The drawing under review shows one solid part. Ordinate dimensions are in mm from its lowest x, y, z. Coordinates: 2 decimals unless noted, no trailing zeros. Order: outer loops, then holes, each group sorted by start corner. A loop starts at its lowest first (then second) coordinate and runs counter-clockwise, first axis right, second up. Notation, with made-up numbers: (60.5, 56.5) - (82.5, 56.5) arc R24 cw to (82.5, 73.5) - close; hole circle Ø7 at (48.25, 41). An arc over 180 degrees is marked (long way). Answer in a Markdown table with one row per item.
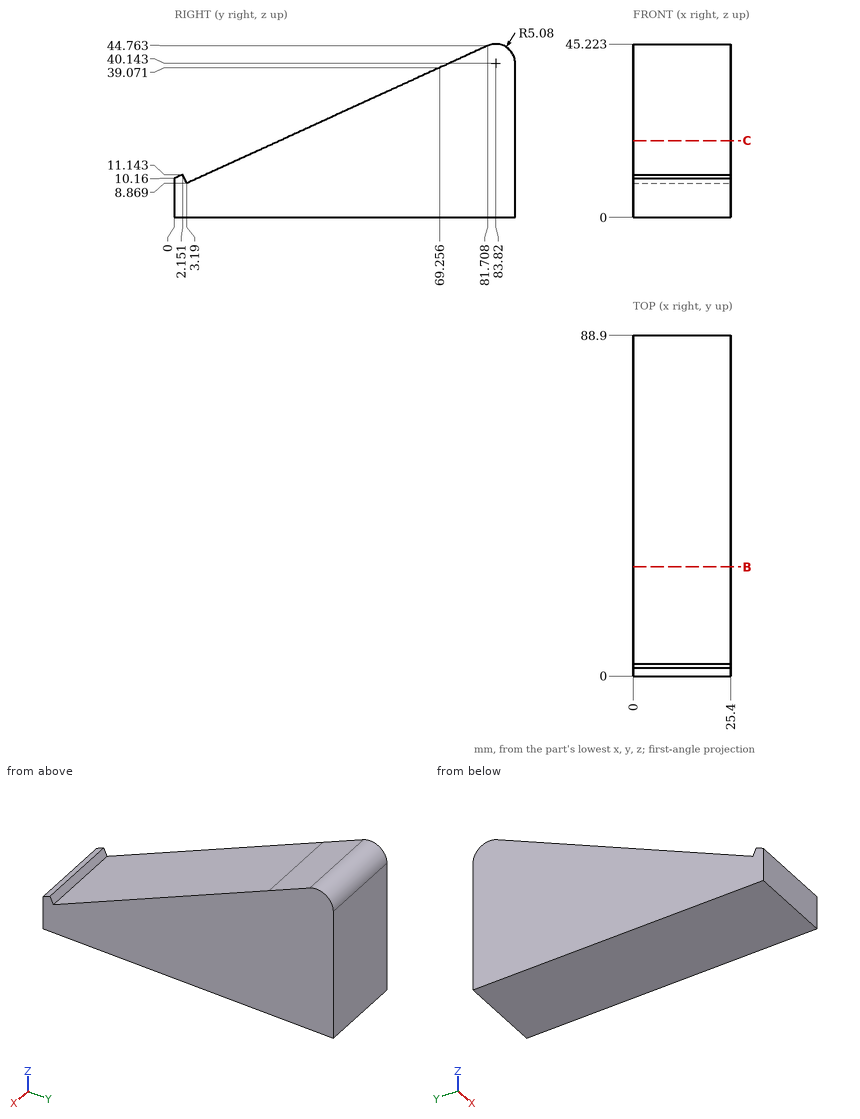
Item 1: We need section C-C, the plane z = 20. Write out the cut boundary in (x, y), then the cut area to 3 significant figures.
Check values:
| item | result |
|---|---|
| outline | (0, 27.54) - (25.4, 27.54) - (25.4, 88.9) - (0, 88.9) - close |
| area | 1,560 mm^2 |
Item 2: To check wall thickness, follow line 1 (Y direction, x = 10.75, z = 10.5) (1 decimal); line 2 (Z direction, x = 21.25, y = 23) (1 decimal); line 3 (Z direction, x = 14.5, y = 16.5) (1 decimal). State the ranges of each line that lie inside material, in increasing order. Write a range as from..to.
Check values:
| item | result |
|---|---|
| line 1 | 0.7..2.4, 6.8..88.9 |
| line 2 | 0..17.9 |
| line 3 | 0..15 |
Item 3: Clearance check with flat-ended pins moving along their axes: pin 1 Ø2 at (x, z) = (20, 31) entering from -Y (1 decimal); pin 2 Ø8 at (x, z) = (5.5, 25) entering from -Y (1 decimal); pin 3 Ø5 at (x, z) = (8.5, 18.5) entering from -Y (1 decimal); pin 4 Ø6 at (x, y) = (11.5, 75.5) entering from -Z. State where each tip first meets the part, or that it passes through.
Check values:
| item | result |
|---|---|
| pin 1 | y = 49.4 |
| pin 2 | y = 29.7 |
| pin 3 | y = 18.8 |
| pin 4 | z = 0 |
Item 4: We need section B-B, the plane y = 28.5. Write out the cut boundary in (x, z).
Check values:
| item | result |
|---|---|
| outline | (0, 0) - (25.4, 0) - (25.4, 20.44) - (0, 20.44) - close |
